Read the model definition and answer for the solid it produces. Units are mm, in the model's axes. Face numbers are marked on the shaded views. Round coordinates to 2 decimals unless told otherwise and drop trailing zeros.
from build123d import *

# Parameters (mm, degrees)
F3_R     = 8.89
F3_R_2   = 5.9436
F5_R     = 7.62
F5_R_2   = 5.9436
F7_DEPTH = 12.7
F6_R     = 7.62
F6_R_2   = 5.9436
F8_DEPTH = 12.7


with BuildPart() as f4:
    # F4: sweep along a path in F2
    with BuildLine(Plane(origin=(0, 0, 0), x_dir=(0.7208469435, 0, -0.6930942822), z_dir=(0.6930942822, 0, 0.7208469435))) as f4_path:
        Line((0, 0), (0, 12.7))
        ThreePointArc((0, 12.7), (35.2363278, 47.9363278), (70.4726556, 12.7))
        Line((70.4726556, 12.7), (70.4726556, 0))
    # F3 (on Front) → F4 (sweep)
    with BuildSketch(Plane.XZ):
        Circle(F3_R)
        Circle(F3_R_2, mode=Mode.SUBTRACT)
    sweep(path=f4_path.line)

    # F5 (on face) → F7 (cut)
    with BuildSketch(Plane.XZ):
        Circle(F5_R)
        Circle(F5_R_2, mode=Mode.SUBTRACT)
    extrude(amount=-F7_DEPTH, mode=Mode.SUBTRACT)

    # F6 (on face) → F8 (cut)
    with BuildSketch(Plane.XZ):
        with Locations((50.7999983902, -48.8441946486)):
            Circle(F6_R)
        with Locations((50.7999983902, -48.8441946486)):
            Circle(F6_R_2, mode=Mode.SUBTRACT)
    extrude(amount=-F8_DEPTH, mode=Mode.SUBTRACT)


solid = f4.part
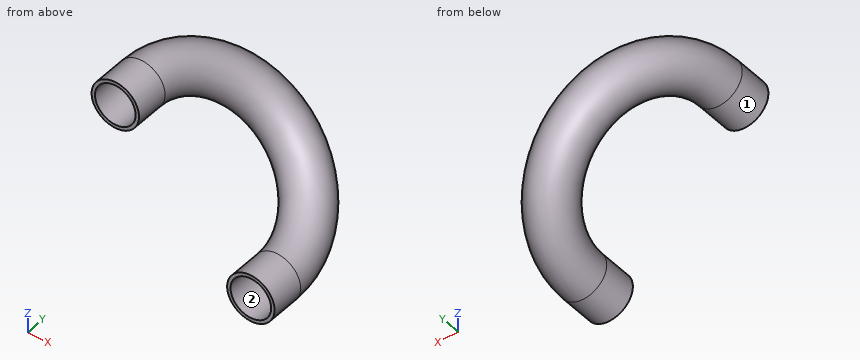
Q1. For a pull along X with two mould halves and no side action, classify the marked faces 1 and 2 as released by +X, released by -X, zero draft, split by the parting line, or undercut.
Outcome:
face 1: split by the parting line
face 2: undercut
Q2. Flat-ended cylindrical pins translate along their axes: pin 1 (2 mm diameter, centred on x = -0.5, y = 11, fed in from -Z); pin 2 (10 mm diameter, centred on y = 31, z = 0.5, fed in from +X); pin 3 (17.5 mm diameter, centred on x = 50.8, z = -48.84, fed in from +Y); pin 4 (17 mm diameter, centred on x = 2, z = 2, fed in from -Y). Find the tip coordinate at first contact, or state that the pin passes through.
Outcome:
pin 1: stops at z = -8.89
pin 2: stops at x = 14.73
pin 3: stops at y = 48
pin 4: stops at y = 0
Q3. Straight lines are drawn through the part: probe 1 along Z at (x, y) = (0, 3.5); probe 2 along X at (y, z) = (12.5, -0.5); probe 3 along X at (y, z) = (39, -43.5). For each, find the intervals that lie inside material, in ascending order.
Outcome:
probe 1: z = -8.89 to -7.62, 7.62 to 8.89
probe 2: x = -8.88 to -7.6, 7.6 to 8.88
probe 3: x = 33.12 to 36.87, 49.55 to 53.02
Q4. A cutting plane is placed at A-A, the plane y = 35.5. Give the number of separate pieces and of enclosed holes in the cut face, plus the area to 3 significant figures.
Outcome:
separate pieces: 2
enclosed holes: 2
area: 381 mm2
